```python
from build123d import *

# Parameters (mm, degrees)
SKETCH_1_W                       = 100
SKETCH_1_H                       = 120
SM_BASE_FLANGE_1_DEPTH           = 3
SM_EDGE_FLANGE_1_STRIP_W         = 13.4732
SM_EDGE_FLANGE_1_STRIP_H         = 3
SM_EDGE_FLANGE_1_STRIP_CUT_DEPTH = 100
SM_EDGE_FLANGE_1_DEPTH           = 100
HOLE_WIZARD_M6_2_D               = 5
HOLE_WIZARD_M6_2_DEPTH           = 15
HOLE_WIZARD_M6_2_CSINK_D         = 6.05
HOLE_WIZARD_M6_2_CSINK_ANGLE     = 90
HOLE_WIZARD_M6_2_TIP             = 1.502151548
HOLE_WIZARD_M8_1_D               = 9
HOLE_WIZARD_M8_1_DEPTH           = 15
HOLE_WIZARD_M8_1_CSINK_D         = 9.05
HOLE_WIZARD_M8_1_CSINK_ANGLE     = 90
HOLE_WIZARD_M8_1_TIP             = 2.703872786


# Sheet-metal steps are written as plain solids
with BuildPart() as part:
    # Sketch 1 → 基体-法兰1 (new body)
    with BuildSketch(Plane.XY):
        Rectangle(SKETCH_1_W, SKETCH_1_H)
    extrude(amount=-SM_BASE_FLANGE_1_DEPTH)

    # 边线-法兰1 strip (across the edge) → 边线-法兰1 strip cut (cut)
    with BuildSketch(Plane(origin=(50, 60, 0), x_dir=(0, -1, 0), z_dir=(-1, 0, 0))):
        with Locations((-3, -1.5)):
            Rectangle(SM_EDGE_FLANGE_1_STRIP_W, SM_EDGE_FLANGE_1_STRIP_H)
    extrude(amount=SM_EDGE_FLANGE_1_STRIP_CUT_DEPTH, mode=Mode.SUBTRACT)

    # 边线-法兰1 section (across the edge) → 边线-法兰1 (add)
    with BuildSketch(Plane(origin=(50, 60, 0), x_dir=(0, -1, 0), z_dir=(-1, 0, 0))):
        with BuildLine():
            Line((0, 0.7366), (0, 57))
            Line((0, 57), (3, 57))
            Line((3, 57), (3, 0.7366))
            ThreePointArc((3, 0.7366), (3.215745145, 0.215745145), (3.7366, 0))
            Line((3.7366, 0), (3.7366, -3))
            ThreePointArc((3.7366, -3), (1.094424801, -1.905575199), (0, 0.7366))
        make_face()
    extrude(amount=SM_EDGE_FLANGE_1_DEPTH)

    # M6 螺纹孔2
    with Locations(Plane(origin=(0, 0, -3), x_dir=(-1, 0, 0), z_dir=(0, 0, -1))):
        with Locations((-36.77, 36.77), (36.77, 36.77), (36.77, -36.77), (-36.77, -36.77)):
            CounterSinkHole(HOLE_WIZARD_M6_2_D / 2, HOLE_WIZARD_M6_2_CSINK_D / 2, depth=HOLE_WIZARD_M6_2_DEPTH, counter_sink_angle=HOLE_WIZARD_M6_2_CSINK_ANGLE)
            with Locations((0, 0, -(HOLE_WIZARD_M6_2_DEPTH + HOLE_WIZARD_M6_2_TIP / 2))):  # 118° drill point
                Cone(0, HOLE_WIZARD_M6_2_D / 2, HOLE_WIZARD_M6_2_TIP, mode=Mode.SUBTRACT)

    # M8 间隙孔1
    with Locations(Plane(origin=(0, 57, 0), x_dir=(-1, 0, 0), z_dir=(0, -1, 0))):
        with Locations((20, -29), (-20, -29)):
            CounterSinkHole(HOLE_WIZARD_M8_1_D / 2, HOLE_WIZARD_M8_1_CSINK_D / 2, depth=HOLE_WIZARD_M8_1_DEPTH, counter_sink_angle=HOLE_WIZARD_M8_1_CSINK_ANGLE)
            with Locations((0, 0, -(HOLE_WIZARD_M8_1_DEPTH + HOLE_WIZARD_M8_1_TIP / 2))):  # 118° drill point
                Cone(0, HOLE_WIZARD_M8_1_D / 2, HOLE_WIZARD_M8_1_TIP, mode=Mode.SUBTRACT)


solid = part.part
```
For this review, take the finished solid that the model builds, in its own axes (mm). A direction names the side the tool comes from. Give positions to 0.01 mm unless a question says otherwise; leave off trailing zeros. Write each loop counter-clockwise with the first axis right and the second up, starting at its lowest first coordinate (ties: lowest second). Pieces come first, ordered by that corner, then holes. Notation, with made-up numbers: M -10.5,-27 L -4.5,-27 A19 cw -4.5,1 Z; hole C 47,-21 d6. An arc over 180 degrees is marked long. Answer as CSV lines item,"result".
1. Consider section C-C, the plane y = 36.77. Write out the cut boundary in (x, z) (3 decimals), then the cut area to 3 significant figures.
Findings:
outline,"M -50,-3 L -39.795,-3 L -39.27,-2.475 L -39.27,0 L -50,0 Z; M -34.27,-2.475 L -33.745,-3 L 33.745,-3 L 34.27,-2.475 L 34.27,0 L -34.27,0 Z; M 39.27,-2.475 L 39.795,-3 L 50,-3 L 50,0 L 39.27,0 Z"
area,"269 mm2"
2. Consider section B-B, the plane x = 20. Write out the cut boundary in (y, z) (3 decimals).
Findings:
outline,"M -60,-3 L 56.263,-3 A3.737 ccw 60,0.737 L 60,24.5 L 57.025,24.5 L 57,24.475 L 57,0.737 A0.737 cw 56.263,0 L -60,0 Z; M 57,33.525 L 57.025,33.5 L 60,33.5 L 60,57 L 57,57 Z"
3. Wall thickness on line 1 (X direction, y = 57.95, z = 29); line 2 (X direction, y = 36.77, z = -1.4); line 3 (Y direction, x = 36.77, z = -1.6): over which ranges is each line inside the solid? List them lowest first.
Findings:
line 1,"x = -50 to -24.5, -15.5 to 15.5, 24.5 to 50"
line 2,"x = -50 to -39.27, -34.27 to 34.27, 39.27 to 50"
line 3,"y = -60 to -39.27, -34.27 to 34.27, 39.27 to 59.18"
4. For pin 1 (5 mm diameter, centred on x = -31, y = 5, fed in from +Z); pin 2 (17 mm diameter, centred on x = 18.5, z = 25.5, fed in from -Y), all flat-tipped, find the tip position at first contact; note any pin that passes through.
Findings:
pin 1,"stops at z = 0"
pin 2,"stops at y = 57"
5. Draft analysis for pull direction Z (two halves, no side actions). For faces 3 (the cylindrical face through (16.4, 58.5, 31.7)), 4 (the cylindrical face through (37.92, 34.55, -1.22)), 5 (the flat face through (-1, -1, 0)), 6 (the cylindrical face through (0.7, 58.88, -1.93)), state which applies: +Z half, -Z half, draft (parallel to the pull), parting line (faces both ways), or undercut.
Findings:
face 3,"undercut"
face 4,"draft"
face 5,"+Z half"
face 6,"-Z half"
6. Consider section D-D, the plane x = 36.77. Write out the cut boundary in (y, z) (3 decimals).
Findings:
outline,"M -60,-3 L -39.795,-3 L -39.27,-2.475 L -39.27,0 L -60,0 Z; M -34.27,-2.475 L -33.745,-3 L 33.745,-3 L 34.27,-2.475 L 34.27,0 L -34.27,0 Z; M 39.27,-2.475 L 39.795,-3 L 56.263,-3 A3.737 ccw 60,0.737 L 60,57 L 57,57 L 57,0.737 A0.737 cw 56.263,0 L 39.27,0 Z"
7. For faces 1 (the flat face through (1, 57, 29)), 2 (the flat face through (1, 59, 57)), list the 3-axis set-ups (+Z, -Z, +X, -X, +Y, -Y) from which the entire face can be reached by the end or side of a thin tool; tool diameter is ignored.
Findings:
face 1,"+Z, +X, -X, -Y"
face 2,"+Z, +X, -X, +Y, -Y"
8. Consider section A-A, the plane z = 29. Write out the cut boundary in (x, y) (3 decimals), then the cut area to 3 significant figures.
Findings:
outline,"M -50,57 L -24.525,57 L -24.5,57.025 L -24.5,60 L -50,60 Z; M -15.5,57.025 L -15.475,57 L 15.475,57 L 15.5,57.025 L 15.5,60 L -15.5,60 Z; M 24.5,57.025 L 24.525,57 L 50,57 L 50,60 L 24.5,60 Z"
area,"246 mm2"
